```python
from build123d import *

# Parameters (mm, degrees)
F0_W     = 70
F0_H     = 35
F0_R     = 4
F0_R_2   = 10.05
F1_DEPTH = 12
F2_R     = 2.1
F3_DEPTH = 15
F4_R     = 2.1
F5_DEPTH = 7.6728517519
F6_SIZE  = 0.5


with BuildPart() as f1:
    # F0 (on Top) → F1 (new body)
    with BuildSketch(Plane.XY):
        with Locations((35, 17.5)):
            Rectangle(F0_W, F0_H)
        with Locations((35, 11.5)):
            Circle(F0_R, mode=Mode.SUBTRACT)
        with Locations((17.5, 17.5)):
            Circle(F0_R_2, mode=Mode.SUBTRACT)
        with Locations((52.5, 17.5)):
            Circle(F0_R_2, mode=Mode.SUBTRACT)
    extrude(amount=F1_DEPTH)

    # F2 (on face) → F3 (cut)
    with BuildSketch(Plane(origin=(0, 35, 0), x_dir=(-1, 0, 0), z_dir=(0, 1, 0))):
        with Locations((-35, 6)):
            Circle(F2_R)
        with Locations((-65, 6)):
            Circle(F2_R)
        with Locations((-5, 6)):
            Circle(F2_R)
    extrude(amount=-F3_DEPTH, mode=Mode.SUBTRACT)

    # F4 (on face) → F5 (cut, through all)
    with BuildSketch(Plane.XZ):
        with Locations((17.5, 6)):
            Circle(F4_R)
        with Locations((52.5, 6)):
            Circle(F4_R)
    extrude(amount=-F5_DEPTH, mode=Mode.SUBTRACT)

    # F6
    f6_edges = [f1.edges().sort_by_distance(p)[0] for p in [
        (31, 11.5, 12),
        (31, 11.5, 0),
    ]]
    chamfer(f6_edges, length=F6_SIZE)


solid = f1.part
```
Here's how the part is built. I have some questions about the finished solid (model axes, mm). A direction names the side the tool comes from. Round coordinates to 2 decimals unless told otherwise and drop trailing zeros. Order: outer loops, then holes, each group sorted by start corner. A loop starts at its lowest first (then second) coordinate and runs counter-clockwise, first axis right, second up. Notation, with made-up numbers: M -0.5,51 L 54.5,51 A29 cw 54.5,85 Z; hole C 56,85.25 d2. An arc over 180 degrees is marked long. Answer in a Markdown table with one row per item.
Item 1: If I drill on L1, parallel to X at y = 10.5, z = 2; L2, parallel to Z at x = 65, y = 31; L3, parallel to X at y = 29, z = 7.5, over which ranges is the centre line in solid material (lowest first)? Write a range as from..to.
A:
| item | result |
|---|---|
| L1 | x = 0..10.29, 24.71..31.13, 38.87..45.29, 59.71..70 |
| L2 | z = 0..3.9, 8.1..12 |
| L3 | x = 0..3.53, 6.47..33.53, 36.47..63.53, 66.47..70 |
Item 2: Imagine slicing it at B-B, the plane z = 8.75. Write out the boundary of the cut face in (x, y).
A:
| item | result |
|---|---|
| outline | M 0,0 L 70,0 L 70,35 L 0,35 Z; hole C 17.5,17.5 d20.1; hole C 35,11.5 d8; hole C 52.5,17.5 d20.1 |
Item 3: Imagine slicing it at D-D, the plane x = 35. Write out the boundary of the cut face in (y, z).
A:
| item | result |
|---|---|
| outline | M 0,0 L 7,0 L 7.5,0.5 L 7.5,11.5 L 7,12 L 0,12 Z; M 15.5,0.5 L 16,0 L 35,0 L 35,3.9 L 20,3.9 L 20,8.1 L 35,8.1 L 35,12 L 16,12 L 15.5,11.5 Z |
Item 4: Imagine slicing it at C-C, the plane y = 23. Write out the boundary of the cut face in (x, z), and give its area (3 significant figures).
A:
| item | result |
|---|---|
| outline | M 0,0 L 9.09,0 L 9.09,12 L 0,12 Z; M 25.91,0 L 44.09,0 L 44.09,12 L 25.91,12 Z; M 60.91,0 L 70,0 L 70,12 L 60.91,12 Z; hole C 5,6 d4.2; hole C 35,6 d4.2; hole C 65,6 d4.2 |
| area | 395 mm2 |
Item 5: Imagine slicing it at A-A, the plane x = 52.5. Write out the boundary of the cut face in (y, z).
A:
| item | result |
|---|---|
| outline | M 0,0 L 7.45,0 L 7.45,3.9 L 0,3.9 Z; M 0,8.1 L 7.45,8.1 L 7.45,12 L 0,12 Z; M 27.55,0 L 35,0 L 35,12 L 27.55,12 Z |
Item 6: Thinking about a two-plate mould opening in Y: for faces 1 (the face through (22.137, 8.584, 5.916)), 2 (the face through (37.1, 27.6, 6.09)), 3 (the face through (5, 20, 6)), which applies, +Y half, -Y half, draft (parallel to the pull), parting line (faces both ways), or undercut?
A:
| item | result |
|---|---|
| face 1 | undercut |
| face 2 | draft |
| face 3 | +Y half |
Item 7: For faces 4 (the face through (19.503, 3.785, 6.631)), 5 (the face through (0, 17, 6)), 6 (the face through (65, 20, 6)), which set-ups out of +Z, -Z, +X, -X, +Y, -Y let a thin tool reach every point of the face, with its end or its side?
A:
| item | result |
|---|---|
| face 4 | -Y |
| face 5 | +Z, -Z, -X, +Y, -Y |
| face 6 | +Y |
Item 8: I'm going to push flat-ended pins straight in: pin 1 (5.5 mm diameter, centred on x = 35, z = 6, fed in from +Y); pin 2 (1.3 mm diameter, centred on x = 65.5, z = 7, fed in from +Y); pin 3 (3 mm diameter, centred on x = 51.5, y = 24.5, fed in from -Z). Where does each tip first touch, or does it pass through?
A:
| item | result |
|---|---|
| pin 1 | stops at y = 35 |
| pin 2 | stops at y = 20 |
| pin 3 | passes through |
